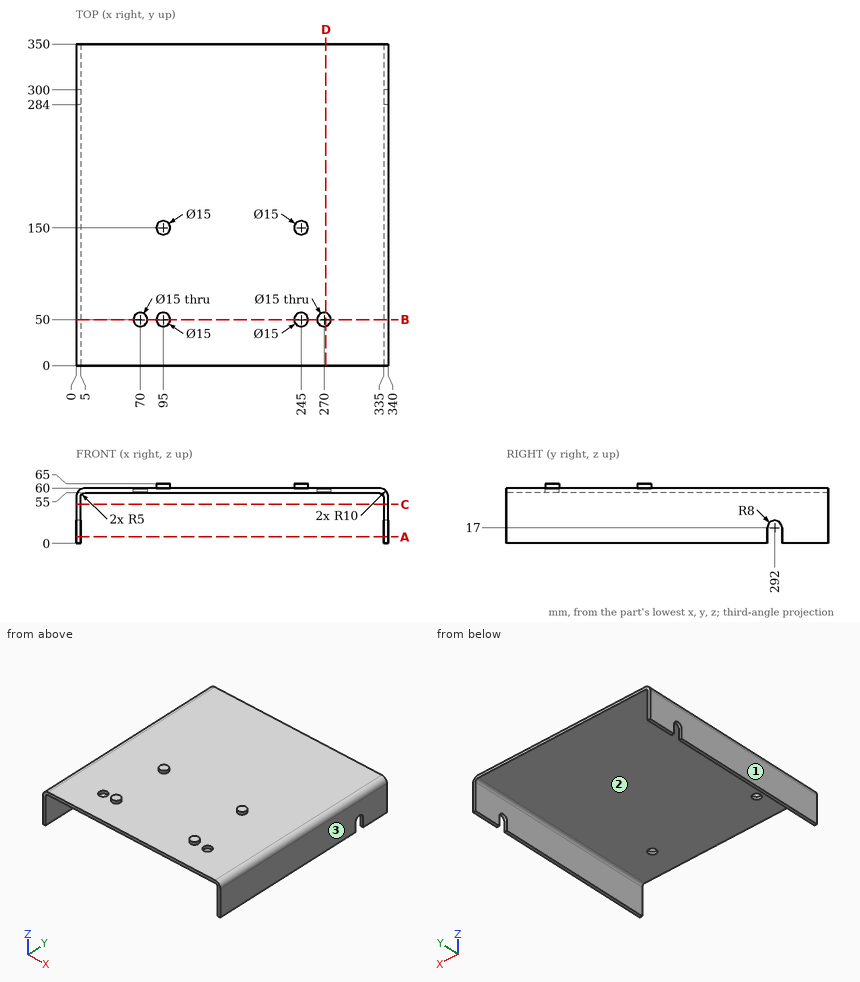
Part print with two shaded views. Sizes in mm from the minimum x, y, z corner. Round coordinates to 2 decimals unless told otherwise and drop trailing zeros. Order: outer loops, then holes, each group sorted by start corner. A loop starts at its lowest first (then second) coordinate and runs counter-clockwise, first axis right, second up. Notation, with made-up numbers: M 22.25,11.25 L 37.25,11.25 A21 ccw 37.25,18.25 Z; hole C 0,-22.75 d2. An arc over 180 degrees is marked long. Use CSV: the item, a comma, the result in double quotes. Start each with the question number.
(1) Drill centre lines: probe 1 along X at (y, z) = (166, 11); probe 2 along X at (y, z) = (50, 56.9); probe 3 along Z at (x, y) = (130.5, 277.5). Where is each one in solid material? Low to high.
(2) Mould opens along X. For the marked faces 1, 2 and 3 say: +X half, -X half, draft (parallel to the pull), parting line (faces both ways), or undercut.
(3) Cut at C-C on z = 42.5. List the corners of the cut face in (x, y), then the cut area to 3 significant figures.
(4) Cut at B-B on y = 50. List the corners of the cut face in (x, z).
(5) Flat gauge pins, fed straight in: P1, Ø1.5, axis at y = 245, z = 57.5, coming from the -X side; P2, Ø4, axis at x = 157.5, y = 303, coming from the +Z side; P3, Ø2, axis at x = 246.5, y = 147.5, coming from the -Z side; P4, Ø1.5, axis at x = 337, z = 5.5, coming from the -Y side. Where does each tip first touch, or does it go through?
(6) Cut at D-D on x = 272. List the corners of the cut face in (y, z), then the cut area to 3 significant figures.
(7) Cut at A-A on z = 7. List the corners of the cut face in (x, y), then the cut area to 3 significant figures.
Findings:
1,probe 1,"x = 0 to 5, 335 to 340"
1,probe 2,"x = 2.76 to 62.5, 77.5 to 262.5, 277.5 to 337.24"
1,probe 3,"z = 55 to 60"
2,face 1,"-X half"
2,face 2,"undercut"
2,face 3,"+X half"
3,outline,"M 0,0 L 5,0 L 5,350 L 0,350 Z; M 335,0 L 340,0 L 340,350 L 335,350 Z"
3,area,"3,500 mm^2"
4,outline,"M 0,0 L 5,0 L 5,50 A5 cw 10,55 L 62.5,55 L 62.5,60 L 10,60 A10 ccw 0,50 Z; M 77.5,55 L 262.5,55 L 262.5,60 L 252.5,60 L 252.5,65 L 237.5,65 L 237.5,60 L 102.5,60 L 102.5,65 L 87.5,65 L 87.5,60 L 77.5,60 Z; M 277.5,55 L 330,55 A5 cw 335,50 L 335,0 L 340,0 L 340,50 A10 ccw 330,60 L 277.5,60 Z"
5,P1,"stops at x = 2.62"
5,P2,"stops at z = 60"
5,P3,"stops at z = 55"
5,P4,"stops at y = 0"
6,outline,"M 0,55 L 42.77,55 L 42.77,60 L 0,60 Z; M 57.23,55 L 350,55 L 350,60 L 57.23,60 Z"
6,area,"1,680 mm^2"
7,outline,"M 0,0 L 5,0 L 5,284 L 0,284 Z; M 0,300 L 5,300 L 5,350 L 0,350 Z; M 335,0 L 340,0 L 340,284 L 335,284 Z; M 335,300 L 340,300 L 340,350 L 335,350 Z"
7,area,"3,340 mm^2"
